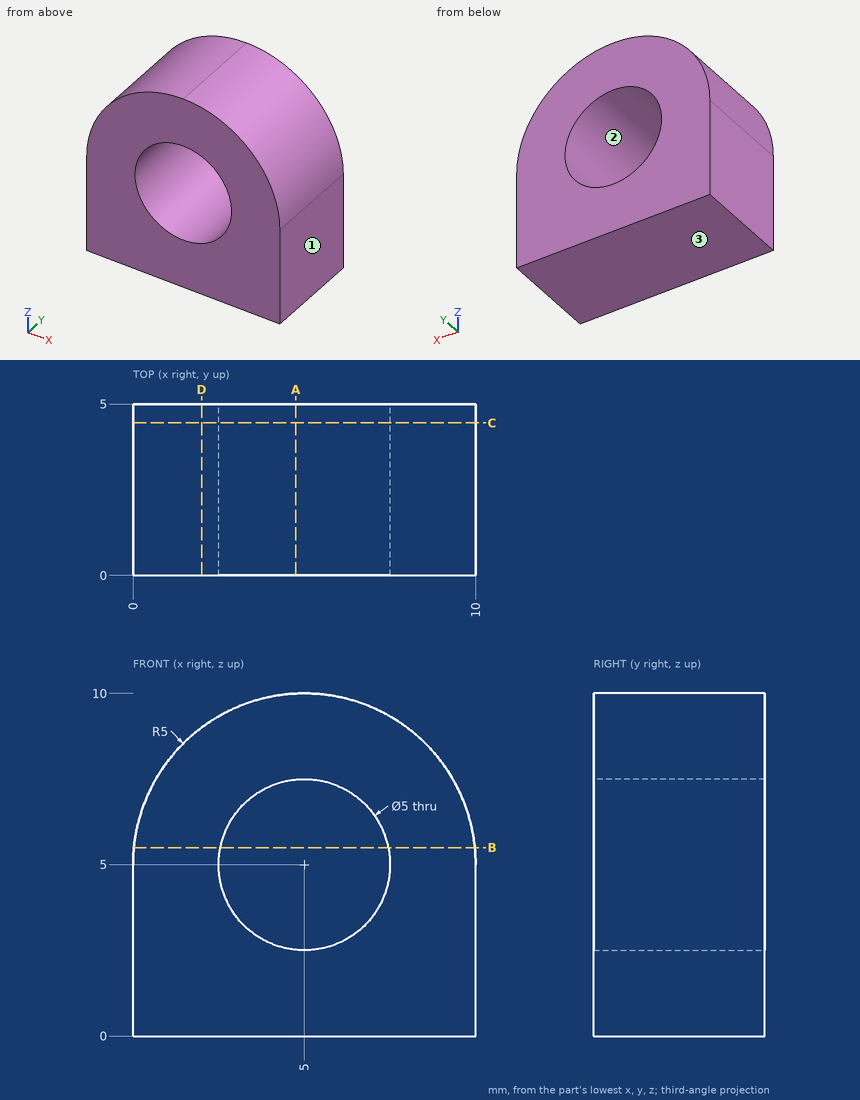
Could you check a few things on this drawing? It's one solid part, dimensions in mm from its lowest x, y, z. Coordinates: 2 decimals unless noted, no trailing zeros. Loops run counter-clockwise (first coordinate to the right, second up) from the corner with the lowest first, then second, coordinate; pieces in that order, holes last.
1. Imagine slicing it at A-A (x = 4.75). Please give me the cut outline in (y, z).
2. Imagine slicing it at D-D (x = 2). Please give me the cut outline in (y, z), and give its area (3 significant figures).
3. I need wall thicknesses on L1, parallel to X at y = 1.75, z = 5; L2, parallel to Z at x = 3.75, y = 2. Which ranges of each line are inside material? Lowest first, please.
4. We'd pull the mould along Z, two halves only. Please class the marked faces 1, 2 and 3: released by +Z, released by -Z, zero draft, split by the parting line, or undercut.
5. Imagine slicing it at B-B (z = 5.5). Please give me the cut outline in (x, y), and give its area (3 significant figures).
6. For P1, Ø4.5, axis at x = 5, z = 5, coming from the +Y side; P2, Ø1, axis at x = 1.5, y = 2, coming from the +Z side; P3, Ø1.5, axis at x = 7.5, y = 1, coming from the +Z side; P4, Ø2, axis at y = 3.5, z = 7, coming from the -X side, each with a flat end and sliding along its axis, tell me the tip position at first contact or that it passes through.
7. Imagine slicing it at C-C (y = 4.45). Please give me the cut outline in (x, z), and give its area (3 significant figures).
Computed values:
1. outline: (0, 0) - (5, 0) - (5, 2.51) - (0, 2.51) - close; (0, 7.49) - (5, 7.49) - (5, 9.99) - (0, 9.99) - close
2. outline: (0, 0) - (5, 0) - (5, 9) - (0, 9) - close
2. area: 45.0 mm2
3. L1: x = 0 to 2.5, 7.5 to 10
3. L2: z = 0 to 2.83, 7.17 to 9.84
4. face 1: zero draft
4. face 2: undercut
4. face 3: released by -Z
5. outline: (0.03, 0) - (2.55, 0) - (2.55, 5) - (0.03, 5) - close; (7.45, 0) - (9.97, 0) - (9.97, 5) - (7.45, 5) - close
5. area: 25.3 mm2
6. P1: passes through
6. P2: stops at z = 9
6. P3: stops at z = 9.68
6. P4: stops at x = 0.1
7. outline: (0, 0) - (10, 0) - (10, 5) arc R5 ccw to (0, 5) - close; hole circle Ø5 at (5, 5)
7. area: 69.6 mm2
